```python
from build123d import *

# Parameters (mm, degrees)
F0_R     = 1.5
F1_DEPTH = 2
F2_DEPTH = 9
F4_DEPTH = 2.5


with BuildPart() as f1:
    # F0 (on Top) → F1 (new body)
    with BuildSketch(Plane.XY):
        with BuildLine():
            Line((-5, -10), (15, -10))
            Line((15, -10), (15, 10))
            Line((15, 10), (-5, 10))
            Line((-5, 10), (-5, 9))
            Line((-5, 9), (-5, 2.25))
            ThreePointArc((-5, 2.25), (-3.40901, 1.59099), (-2.75, 0))
            ThreePointArc((-2.75, 0), (-3.40901, -1.59099), (-5, -2.25))
            Line((-5, -2.25), (-5, -9))
            Line((-5, -9), (-5, -10))
        make_face()
        with Locations((5, 0)):
            Circle(F0_R, mode=Mode.SUBTRACT)
        with BuildLine():
            ThreePointArc((-15, 0), (-12.071068, -7.071068), (-5, -10))
            Line((-5, -10), (-5, -9))
            ThreePointArc((-5, -9), (-11.363961, -6.363961), (-14, 0))
            ThreePointArc((-14, 0), (-11.363961, 6.363961), (-5, 9))
            Line((-5, 9), (-5, 10))
            ThreePointArc((-5, 10), (-12.071068, 7.071068), (-15, 0))
        make_face()
        with BuildLine():
            ThreePointArc((-14, 0), (-11.363961, -6.363961), (-5, -9))
            Line((-5, -9), (-5, -2.25))
            ThreePointArc((-5, -2.25), (-7.25, 0), (-5, 2.25))
            Line((-5, 2.25), (-5, 9))
            ThreePointArc((-5, 9), (-11.363961, 6.363961), (-14, 0))
        make_face()
    extrude(amount=-F1_DEPTH)

    # F0 (on Top) → F2 (join)
    with BuildSketch(Plane.XY):
        with BuildLine():
            ThreePointArc((-14, 0), (-11.363961, -6.363961), (-5, -9))
            Line((-5, -9), (-5, -2.25))
            ThreePointArc((-5, -2.25), (-7.25, 0), (-5, 2.25))
            Line((-5, 2.25), (-5, 9))
            ThreePointArc((-5, 9), (-11.363961, 6.363961), (-14, 0))
        make_face()
        with BuildLine():
            ThreePointArc((-15, 0), (-12.071068, -7.071068), (-5, -10))
            Line((-5, -10), (-5, -9))
            ThreePointArc((-5, -9), (-11.363961, -6.363961), (-14, 0))
            ThreePointArc((-14, 0), (-11.363961, 6.363961), (-5, 9))
            Line((-5, 9), (-5, 10))
            ThreePointArc((-5, 10), (-12.071068, 7.071068), (-15, 0))
        make_face()
    extrude(amount=F2_DEPTH)

    # F3 (on face) → F4 (join)
    with BuildSketch(Plane.XY.offset(9)):
        with BuildLine():
            Line((-5, 9), (-5, 10))
            ThreePointArc((-5, 10), (-12.071068, 7.071068), (-15, 0))
            ThreePointArc((-15, 0), (-12.071068, -7.071068), (-5, -10))
            Line((-5, -10), (-5, -9))
            ThreePointArc((-5, -9), (-11.363961, -6.363961), (-14, 0))
            ThreePointArc((-14, 0), (-11.363961, 6.363961), (-5, 9))
        make_face()
    extrude(amount=F4_DEPTH)


solid = f1.part
```
Check sheet for the modelled part. Datum: model origin and axes. Units: mm. A direction names the side the tool comes from. Coordinates: 2 decimals unless noted, no trailing zeros. Write each loop counter-clockwise with the first axis right and the second up, starting at its lowest first coordinate (ties: lowest second). Pieces come first, ordered by that corner, then holes. Notation, with made-up numbers: M 31.5,71 L 77.5,71 A5 ccw 77.5,77 Z; hole C 29,21.25 d4. An arc over 180 degrees is marked long. Write item = value, one per line. Start each with the question number.
1. Tool access check on faces 4 (the flat face through (-10, 0, 9)), 5 (the flat face through (-5, -6, 4)), 6 (the flat face through (5, -10, -1)). Record the directions out of +Z, -Z, +X, -X, +Y, -Y that give a thin tool (end or side, any length) a straight path to the whole face; none if there is none.
2. Sectioned sample at C-C (y = 4.75). Record the cut outline in (x, z), then the cut area to 3 significant figures.
3. Mould release check, pull along X, two halves, no side actions. Record for faces 1 (the flat face through (7, 0, 0)), 2 (the cylindrical face through (6.386, -0.575, -0.986)), 3 (the flat face through (-5, 6, 4)): pulls with the +X half, pulls with the -X half, needs draft (parallel to the pull), parting line crosses it, or undercut.
4. Sectioned sample at A-A (x = 5). Record the cut outline in (y, z).
5. Thickness scan on probe 1 along Y at (x, z) = (5, -0.7); probe 2 along Z at (x, y) = (-11.5, -3.5); probe 3 along Z at (x, y) = (5, 7.75). Record the ranges inside material, lowest first.
6. Sectioned sample at B-B (z = 3.25). Record the cut outline in (x, y), then the cut area to 3 significant figures.
7. Sectioned sample at D-D (x = 10). Record the cut outline in (y, z), then the cut area to 3 significant figures.
8. Go/stop test with flat-tipped pins: pin 1 (6 mm diameter, centred on y = 8, z = 7.5, fed in from +X); pin 2 (10 mm diameter, centred on x = -7.5, y = 1.5, fed in from +Z); pin 3 (4 mm diameter, centred on x = 2, y = -2, fed in from +Z). Record where each tip stops, or that it passes through.
The answers:
q1.face_4 = +Z, +X
q1.face_5 = +Z, +X, +Y, -Y
q1.face_6 = +Z, -Z, +X, -X, -Y
q2.outline = M -13.8,-2 L 15,-2 L 15,0 L -5,0 L -5,9 L -12.64,9 L -12.64,11.5 L -13.8,11.5 Z
q2.area = 140 mm²
q3.face_1 = needs draft
q3.face_2 = undercut
q3.face_3 = pulls with the +X half
q4.outline = M -10,-2 L -1.5,-2 L -1.5,0 L -10,0 Z; M 1.5,-2 L 10,-2 L 10,0 L 1.5,0 Z
q5.probe_1 = -10 to -1.5, 1.5 to 10
q5.probe_2 = -2 to 9
q5.probe_3 = -2 to 0
q6.outline = M -15,0 A10 ccw -5,-10 L -5,-2.25 A2.25 cw -5,2.25 L -5,10 A10 ccw Z
q6.area = 149 mm²
q7.outline = M -10,-2 L 10,-2 L 10,0 L -10,0 Z
q7.area = 40.0 mm²
q8.pin_1 = -5
q8.pin_2 = 9
q8.pin_3 = 0
